Source: CAD feature listing. Evaluate the final solid. Frame: model axes, mm. A direction names the side the tool comes from. Coordinates: 2 decimals unless noted, no trailing zeros. Loops run counter-clockwise (first coordinate to the right, second up) from the corner with the lowest first, then second, coordinate; pieces in that order, holes last. Notation, with made-up numbers: (-30.75, 88.5) -> (2.25, 88.5) arc R35 cw to (2.25, 124.5) -> close; hole circle Ø6 at (-7, 31.25). An arc over 180 degrees is marked (long way). Answer as CSV lines item,"result".
from build123d import *

# Parameters (mm, degrees)
RESSALTO_EXTRUS_O1_DEPTH = 25
ESBO_O2_R                = 8
CORTE_EXTRUS_O2_DEPTH    = 9


with BuildPart() as part:
    # Esboço1 → Ressalto-extrusão1 (new body)
    with BuildSketch(Plane(origin=(0, 0, 0), x_dir=(1, 0, 0), z_dir=(0, 1, 0))):
        Polygon((-17.666653224, -22.560793644), (-17.666653224, 0), (-17.666653224, 47.439206356), (2.333346776, 47.439206356), (22.333346776, 47.439206356), (22.333346776, 0), (22.333346776, -22.560793644), (2.333346776, -22.560793644), align=None)
        with BuildLine():
            ThreePointArc((2.333346776, 67.439206356), (16.4754824, 61.581341979), (22.333346776, 47.439206356))
            Line((22.333346776, 47.439206356), (2.333346776, 47.439206356))
            Line((2.333346776, 47.439206356), (2.333346776, 67.439206356))
        make_face()
        with BuildLine():
            Line((2.333346776, 47.439206356), (2.333346776, 67.439206356))
            ThreePointArc((2.333346776, 67.439206356), (-11.808788848, 61.581341979), (-17.666653224, 47.439206356))
            Line((-17.666653224, 47.439206356), (2.333346776, 47.439206356))
        make_face()
    extrude(amount=RESSALTO_EXTRUS_O1_DEPTH)

    # Esboço2 → Corte-extrusão2 (cut)
    with BuildSketch(Plane(origin=(0, 0, 0), x_dir=(1, 0, 0), z_dir=(0, 1, 0))):
        with BuildLine():
            Line((-12.666653224, -22.560793644), (-12.666653224, -9.110478183))
            ThreePointArc((-12.666653224, -9.110478183), (2.333346776, 5.889521817), (17.333346776, -9.110478183))
            Line((17.333346776, -9.110478183), (17.333346776, -22.560793644))
            Line((17.333346776, -22.560793644), (-12.666653224, -22.560793644))
        make_face()
        with Locations(Location((2.333346776, -9.110478183, 0), (0, 0, 270))):
            Circle(ESBO_O2_R, mode=Mode.SUBTRACT)
    extrude(amount=CORTE_EXTRUS_O2_DEPTH, mode=Mode.SUBTRACT)


solid = part.part
(1) Cut plane A-A (y = 7.25). Return the cut outline in (x, z).
Computed values:
outline,"(-17.67, -47.44) arc R20 ccw to (22.33, -47.44) -> (22.33, 22.56) -> (17.33, 22.56) -> (17.33, 9.11) arc R15 cw to (-12.67, 9.11) -> (-12.67, 22.56) -> (-17.67, 22.56) -> close; circle Ø16 at (2.33, 9.11)"
(2) Cut plane D-D (y = 19). Return the cut outline in (x, z), then the cut area to 3 significant figures.
Computed values:
outline,"(-17.67, -47.44) arc R20 ccw to (22.33, -47.44) -> (22.33, 22.56) -> (-17.67, 22.56) -> close"
area,"3,430 mm^2"
(3) Draft query along Z for faces 4 (the cylindrical face through (2.69, 4.44, 1.12)), 5 (the flat face through (17.333, 4, 16)), 6 (the flat face through (2, 15, 22.561)). Return one class per face: released by +Z, released by -Z, zero draft, split by the parting line, or undercut.
Computed values:
face 4,"undercut"
face 5,"zero draft"
face 6,"released by +Z"
(4) Pin query (flat end, axial travel): pin 1 Ø2 at (x, z) = (-4.5, -13.5) entering from -Y; pin 2 Ø6 at (x, y) = (-9, 7.5) entering from -Z. Return the tip coordinate at first contact, or that it passes through.
Computed values:
pin 1,"y = 0"
pin 2,"z = -65.62"
(5) Cut plane B-B (x = 8.5). Return the cut outline in (y, z), then the cut area to 3 significant figures.
Computed values:
outline,"(0, -66.46) -> (25, -66.46) -> (25, 22.56) -> (9, 22.56) -> (9, 14.21) -> (0, 14.21) -> (0, 4.01) -> (9, 4.01) -> (9, -4.56) -> (0, -4.56) -> close"
area,"2,070 mm^2"
(6) Access query for faces 1 (the flat face through (3, 9, 18)), 2 (the flat face through (-12.667, 4, 16)), 3 (the flat face through (2, 0, 9)). Directions: +Z, -Z, +X, -X, +Y, -Y. A direction counts if a zero-diameter tool reaches every point of the face in a straight line with its end or side. Return the directions, or none.
Computed values:
face 1,"-Y"
face 2,"+Z, -Y"
face 3,"+Z, -Z, +X, -X, -Y"
(7) Material intervals for L1, parallel to X at y = 7.25, z = 18; L2, parallel to Y at x = 14.5, z = 16; L3, parallel to Z at x = -3, y = 2.75, sorted ascending. Write a range as [from, to].
Computed values:
L1,"[-17.67, -12.67], [17.33, 22.33]"
L2,"[9, 25]"
L3,"[-66.71, -4.91], [3.15, 15.07]"
(8) Cut plane C-C (z = 3.5). Return the cut outline in (x, y).
Computed values:
outline,"(-17.67, 0) -> (-11.58, 0) -> (-11.58, 9) -> (-3.37, 9) -> (-3.37, 0) -> (8.04, 0) -> (8.04, 9) -> (16.24, 9) -> (16.24, 0) -> (22.33, 0) -> (22.33, 25) -> (-17.67, 25) -> close"
